```python
from build123d import *

# Parameters (mm, degrees)
F0_R      = 26.75
F0_R_2    = 21.75
F1_DEPTH  = 25
F3_R      = 22.935905
F3_R_2    = 18.75
F4_DEPTH  = 2
F6_R      = 35
F7_R      = 26.75
F9_R      = 30
F10_R     = 18.714906
F12_R     = 35
F12_R_2   = 30
F13_DEPTH = 25
F16_DEPTH = 5.2


with BuildPart() as f1:
    # F0 (on Top) → F1 (new body)
    with BuildSketch(Plane.XY):
        Circle(F0_R)
        Circle(F0_R_2, mode=Mode.SUBTRACT)
    extrude(amount=F1_DEPTH)

    # F3 (on offset) → F4 (join)
    with BuildSketch(Plane.XY.offset(11.9)):
        Circle(F3_R)
        Circle(F3_R_2, mode=Mode.SUBTRACT)
    extrude(amount=F4_DEPTH)

    # F6 (on offset) → F8 section 0
    with BuildSketch(Plane.XY.offset(50)):
        Circle(F6_R)
    # F7 (on face) → F8 section 1
    with BuildSketch(Plane.XY.offset(25)):
        Circle(F7_R)
    loft()

    # F9 (on face) → F11 section 0
    with BuildSketch(Plane.XY.offset(50)):
        Circle(F9_R)
    # F10 (on face) → F11 section 1
    with BuildSketch(Plane(origin=(0, 0, 11.9), x_dir=(1, 0, 0), z_dir=(0, 0, -1))):
        Circle(F10_R)
    loft(mode=Mode.SUBTRACT)

    # F12 (on face) → F13 (join)
    with BuildSketch(Plane.XY.offset(50)):
        Circle(F12_R)
        Circle(F12_R_2, mode=Mode.SUBTRACT)
    extrude(amount=F13_DEPTH)

    # F15 (on offset) → F16 (cut)
    with BuildSketch(Plane.XY.offset(60)):
        with BuildLine():
            Line((-0.026878, 29.999988), (-3.897005, 34.782371))
            ThreePointArc((-3.897005, 34.782371), (-35, 0), (-3.897005, -34.782371))
            Line((-3.897005, -34.782371), (-0.026878, -29.999988))
            ThreePointArc((-0.026878, -29.999988), (-30, 0), (-0.026878, 29.999988))
        make_face()
        with BuildLine():
            Line((-0.026878, -29.999988), (-0.026878, 29.999988))
            ThreePointArc((-0.026878, 29.999988), (-30, 0), (-0.026878, -29.999988))
        make_face()
    extrude(amount=F16_DEPTH, mode=Mode.SUBTRACT)


solid = f1.part
```
Here's how the part is built. I have some questions about the finished solid (model axes, mm). A direction names the side the tool comes from. Give positions to 0.01 mm unless a question says otherwise; leave off trailing zeros. Write each loop counter-clockwise with the first axis right and the second up, starting at its lowest first coordinate (ties: lowest second). Pieces come first, ordered by that corner, then holes.
(1) If I drill on L1, parallel to Y at x = 1, z = 5.5; L2, parallel to Y at x = 0, z = 60, over which ranges is the centre line in solid material (lowest first)?
Output values:
L1: y = -26.73 to -21.73, 21.73 to 26.73
L2: y = -35 to -30, 30 to 35
(2) Imagine slicing it at A-A, the plane z = 70.5. Write out the boundary of the cut face in (x, y), and give its area (3 significant figures).
Output values:
outline: circle Ø70 at (0, 0); hole circle Ø60 at (0, 0)
area: 1,020 mm2
(3) Thinking about a two-plate mould opening in Y: for faces 5 (the face through (-5.799, -26.114, 12.325)), 6 (the face through (26, 16, 75)), 7 (the face through (6, 18, 11.9)), which applies, pulls with the +Y half, pulls with the -Y half, needs draft (parallel to the pull), parting line crosses it, or undercut?
Output values:
face 5: parting line crosses it
face 6: needs draft
face 7: undercut
(4) Will these pins go through, and if not, where does the flat tip stop? pin 1 (5 mm diameter, centred on y = -13.5, z = 23.5, fed in from +X); pin 2 (2 mm diameter, centred on y = -21.5, z = 14.5, fed in from +X); pin 3 (1 mm diameter, centred on y = 14, z = 10, fed in from +X).
Output values:
pin 1: stops at x = 24.38
pin 2: stops at x = 17.18
pin 3: stops at x = 23.09
(5) On a 3-axis mill with a long thin cutter (end or side, diameter ignored), from which of +Z, -Z, +X, -X, +Y, -Y can I reach the whole of each face in a straight line? I mean faces 1 (the face through (-2.831, 21.565, 17.966)), 2 (the face through (0, 22, 0)), 3 (the face through (-2.831, 21.565, 5.867)), 4 (the face through (-1.935, 32.358, 62.564)). Say none if no direction works.
Output values:
face 1: +Z
face 2: -Z, +X, -X, +Y, -Y
face 3: -Z
face 4: -X
(6) Imagine slicing it at B-B, the plane y = 0. Count the separate pieces of the cut face and the enclosed holes in it, and give its area (3 significant figures).
Output values:
separate pieces: 3
enclosed holes: 0
area: 711 mm2
(7) Imagine slicing it at D-D, the plane z = 62. Write out the boundary of the cut face in (x, y).
Output values:
outline: (-3.9, -34.78) arc R35 ccw (long way) to (-3.9, 34.78) - (-0.03, 30) arc R30 cw to (-0.03, -30) - close
